Check sheet for the drawn part. Datum: minimum x, y, z corner. Units: mm. Round coordinates to 2 decimals unless told otherwise and drop trailing zeros. Write each loop counter-clockwise with the first axis right and the second up, starting at its lowest first coordinate (ties: lowest second). Pieces come first, ordered by that corner, then holes. Notation, with made-up numbers: (50.25, -16) -> (67.25, -16) arc R30 cw to (67.25, 17) -> close; hole circle Ø6 at (87.5, -34). An arc over 180 degrees is marked (long way). Use CSV: the item, a comma, the result in double quotes.
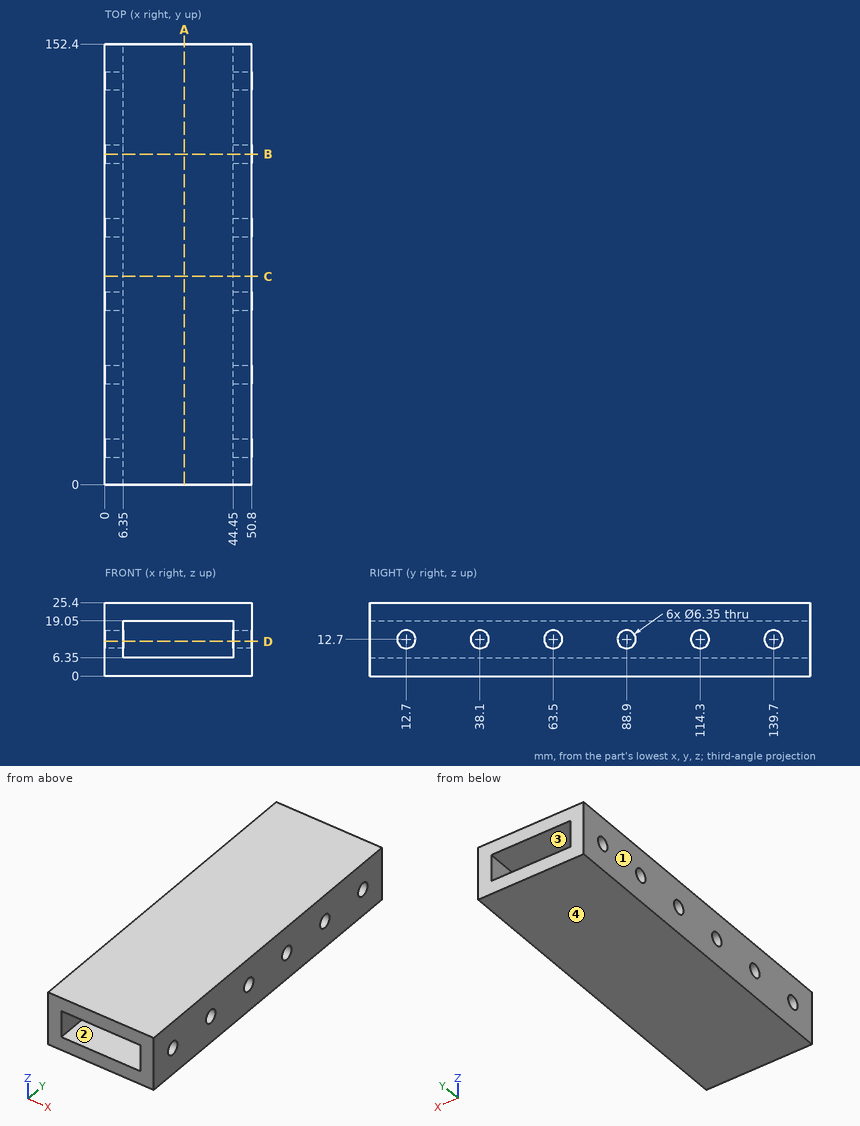
Q1. Section check A-A (x = 27.5). Record the cut outline in (y, z).
Filled in:
outline,"(0, 0) -> (152.4, 0) -> (152.4, 6.35) -> (0, 6.35) -> close; (0, 19.05) -> (152.4, 19.05) -> (152.4, 25.4) -> (0, 25.4) -> close"
Q2. Material ranges on L1, parallel to X at y = 9, z = 7.5; L2, parallel to Z at x = 23.5, y = 138.5; L3, parallel to Z at x = 46, y = 41, recorded low to high.
Filled in:
L1,"0 to 6.35, 44.45 to 50.8"
L2,"0 to 6.35, 19.05 to 25.4"
L3,"0 to 11.41, 13.99 to 25.4"
Q3. Section check D-D (z = 12). State how many separate pieces and enclosed holes the cut face has, plus the area to 3 significant figures.
Filled in:
separate pieces,"14"
enclosed holes,"0"
area,"1,460 mm²"
Q4. Section check C-C (y = 72). Record the cut outline in (x, z), plus the area to 3 significant figures.
Filled in:
outline,"(0, 0) -> (50.8, 0) -> (50.8, 25.4) -> (0, 25.4) -> close; hole (6.35, 6.35) -> (44.45, 6.35) -> (44.45, 19.05) -> (6.35, 19.05) -> close"
area,"806 mm²"
Q5. Mould release check, pull along Z, two halves, no side actions. Record for the marked faces 1, 2, 3 and 4: released by +Z, released by -Z, zero draft, split by the parting line, or undercut.
Filled in:
face 1,"zero draft"
face 2,"undercut"
face 3,"undercut"
face 4,"released by -Z"
Q6. Section check B-B (y = 114.3). Record the cut outline in (x, z) (3 decimals).
Filled in:
outline,"(0, 0) -> (50.8, 0) -> (50.8, 9.525) -> (44.45, 9.525) -> (44.45, 6.35) -> (6.35, 6.35) -> (6.35, 9.525) -> (0, 9.525) -> close; (0, 15.875) -> (6.35, 15.875) -> (6.35, 19.05) -> (44.45, 19.05) -> (44.45, 15.875) -> (50.8, 15.875) -> (50.8, 25.4) -> (0, 25.4) -> close"
